Could you check a few things on this model? Use its own coordinates, in mm. Give positions to 0.01 mm unless a question says otherwise; leave off trailing zeros. Order: outer loops, then holes, each group sorted by start corner. A loop starts at its lowest first (then second) coordinate and runs counter-clockwise, first axis right, second up. Notation, with made-up numbers: (34.25, -26.5) -> (64.25, -26.5) arc R21 cw to (64.25, 0.5) -> close; hole circle Ø2 at (0, 75.25). An arc over 180 degrees is marked (long way). Use one line per item in the form item = value. Start each with the question number.
from build123d import *

# Parameters (mm, degrees)
F0_W     = 300
F0_H     = 180
F0_R     = 10
F1_DEPTH = 25
F2_SIZE  = 2


with BuildPart() as f1:
    # F0 (on Top) → F1 (new body)
    with BuildSketch(Plane.XY):
        Rectangle(F0_W, F0_H)
        with Locations((-121.507466, -65)):
            Circle(F0_R, mode=Mode.SUBTRACT)
        with Locations((0, -65)):
            Circle(F0_R, mode=Mode.SUBTRACT)
        with Locations((128.492534, -65)):
            Circle(F0_R, mode=Mode.SUBTRACT)
        with Locations((-121.507466, 65)):
            Circle(F0_R, mode=Mode.SUBTRACT)
        with Locations((0, 65)):
            Circle(F0_R, mode=Mode.SUBTRACT)
        with Locations((128.492534, 65)):
            Circle(F0_R, mode=Mode.SUBTRACT)
    extrude(amount=F1_DEPTH)

    # F2
    f2_edges = [f1.edges().sort_by_distance(p)[0] for p in [
        (150, 0, 25),
        (0, 90, 25),
        (-150, 0, 25),
        (0, -90, 25),
        (-131.507466, -65, 25),
        (-10, -65, 25),
        (118.492534, -65, 25),
        (-131.507466, 65, 25),
        (-10, 65, 25),
        (118.492534, 65, 25),
        (150, 0, 0),
        (0, 90, 0),
        (-150, 0, 0),
        (0, -90, 0),
        (-131.507466, -65, 0),
        (-10, -65, 0),
        (118.492534, -65, 0),
        (-131.507466, 65, 0),
        (-10, 65, 0),
        (118.492534, 65, 0),
    ]]
    chamfer(f2_edges, length=F2_SIZE)


solid = f1.part
(1) Please list where these lines run through material, in increasing order: probe 1 along X at (y, z) = (72, 9.75); probe 2 along Y at (x, z) = (-7.5, 3); probe 3 along Y at (x, z) = (-44, 1.5).
(2) Imagine slicing it at A-A (x = 0). Write out the boundary of the cut face in (y, z), plus the area to 3 significant figures.
(3) Imagine slicing it at C-C (z = 16). Write out the boundary of the cut face in (x, y), plus the area to 3 significant figures.
(4) Imagine slicing it at B-B (y = 65). Give the number of separate pieces and of enclosed holes in the cut face, plus the area to 3 significant figures.
(5) We'd pull the mould along X, two halves only. Please class faces 1 (the flat face through (150, -1, 12)), 2 (the flat face through (-150, -1, 12)), 3 (the conical face through (-1.318, -54.961, 23.125)), 4 (the flat face through (-2, 1, 25)): pulls with the +X half, pulls with the -X half, needs draft (parallel to the pull), parting line crosses it, or undercut.
Calculated:
q1.probe_1 = -150 to -128.65, -114.37 to -7.14, 7.14 to 121.35, 135.63 to 150
q1.probe_2 = -90 to -71.61, -58.39 to 58.39, 71.61 to 90
q1.probe_3 = -89.5 to 89.5
q2.outline = (-90, 2) -> (-88, 0) -> (-77, 0) -> (-75, 2) -> (-75, 23) -> (-77, 25) -> (-88, 25) -> (-90, 23) -> close; (-55, 2) -> (-53, 0) -> (53, 0) -> (55, 2) -> (55, 23) -> (53, 25) -> (-53, 25) -> (-55, 23) -> close; (75, 2) -> (77, 0) -> (88, 0) -> (90, 2) -> (90, 23) -> (88, 25) -> (77, 25) -> (75, 23) -> close
q2.area = 3,480 mm2
q3.outline = (-150, -90) -> (150, -90) -> (150, 90) -> (-150, 90) -> close; hole circle Ø20 at (-121.51, -65); hole circle Ø20 at (-121.51, 65); hole circle Ø20 at (0, -65); hole circle Ø20 at (0, 65); hole circle Ø20 at (128.49, -65); hole circle Ø20 at (128.49, 65)
q3.area = 52,100 mm2
q4.separate_pieces = 4
q4.enclosed_holes = 0
q4.area = 5,970 mm2
q5.face_1 = pulls with the +X half
q5.face_2 = pulls with the -X half
q5.face_3 = undercut
q5.face_4 = needs draft
